Input: part model. Units: mm. Frame: model coordinates. A direction names the side the tool comes from. Coordinates: 2 decimals unless noted, no trailing zeros. Write each loop counter-clockwise with the first axis right and the second up, starting at its lowest first coordinate (ties: lowest second). Pieces come first, ordered by that corner, then holes. Notation, with made-up numbers: M 55,9.25 L 81,9.25 A28 cw 81,40.25 Z; hole C 53.25,70.25 d1. An arc over 180 degrees is marked long. Use one line per item in the form item = value.
from build123d import *

# Parameters (mm, degrees)
BOSS_EXTRUDE1_DEPTH = 100
CUT_EXTRUDE3_REACH  = 138.159
FILLET2_R           = 20
SKETCH6_R           = 4
CUT_EXTRUDE4_DEPTH  = 15


with BuildPart() as part:
    # Sketch1 → Boss-Extrude1 (new body)
    with BuildSketch(Plane.YZ):
        with BuildLine():
            Line((-12.5, 0), (-12.5, -8))
            Line((-12.5, -8), (-10.019077862, -8))
            ThreePointArc((-10.019077862, -8), (-7.561621729, -9.279270691), (-7.2, -12.02606043))
            Line((-7.2, -12.02606043), (-32.25, -80.850369787))
            Line((-32.25, -80.850369787), (-18.415688958, -80.850369787))
            Line((-18.415688958, -80.850369787), (7.381221952, -9.97393957))
            ThreePointArc((7.381221952, -9.97393957), (8.479570506, -8.542543867), (10.200299815, -8))
            Line((10.200299815, -8), (12.5, -8))
            Line((12.5, -8), (12.5, 0))
            Line((12.5, 0), (-12.5, 0))
        make_face()
    extrude(amount=-BOSS_EXTRUDE1_DEPTH)

    # Cut-Extrude3: up to this plane
    cut_extrude3_end = Plane(origin=(-100, -7.2, -12.02606043), z_dir=(0, -0.9396926207859074, 0.34202014332567165))
    # Sketch5 → Cut-Extrude3 (cut, up to the surface)
    with BuildSketch(Plane(origin=(0, 12.5, 0), x_dir=(-1, 0, 0), z_dir=(0, 1, 0)), mode=Mode.PRIVATE) as cut_extrude3_sk1:
        with BuildLine():
            Line((10, -15), (10, -60.850369787))
            ThreePointArc((10, -60.850369787), (12.928932188, -67.921437599), (20, -70.850369787))
            Line((20, -70.850369787), (80, -70.850369787))
            ThreePointArc((80, -70.850369787), (87.071067812, -67.921437599), (90, -60.850369787))
            Line((90, -60.850369787), (90, -15))
            Line((90, -15), (10, -15))
        make_face()
    cut_extrude3_tool1 = split(extrude(cut_extrude3_sk1.sketch, amount=-CUT_EXTRUDE3_REACH, mode=Mode.PRIVATE), bisect_by=cut_extrude3_end, keep=Keep.BOTH, mode=Mode.PRIVATE)
    add(cut_extrude3_tool1.solids().sort_by_distance((-50, 12.5, -42.675996))[0], mode=Mode.SUBTRACT)

    # Fillet2
    fillet2_edges = [part.edges().sort_by_distance(p)[0] for p in [
        (0, -25.332844479, -80.850369787),
        (-100, -25.332844479, -80.850369787),
    ]]
    fillet(fillet2_edges, radius=FILLET2_R)

    # Sketch6 → Cut-Extrude4 (cut)
    with BuildSketch(Plane.XY):
        with Locations((-75, 0)):
            Circle(SKETCH6_R)
        with Locations((-25, 0)):
            Circle(SKETCH6_R)
    extrude(amount=-CUT_EXTRUDE4_DEPTH, mode=Mode.SUBTRACT)


solid = part.part
(1) Pull-direction query (Y, two-part tool) for faces 1 (the flat face through (-49, -11, -8)), 2 (the cylindrical face through (-79, 0, -7)), 3 (the cylindrical face through (-28.2, -2.4, -7.4)), 4 (the cylindrical face through (-49.3, 8.459, -8.557)); classes: pulls with the +Y half, pulls with the -Y half, needs draft (parallel to the pull), parting line crosses it, or undercut.
Computed:
face_1 = needs draft
face_2 = undercut
face_3 = undercut
face_4 = pulls with the +Y half
(2) Section query B-B on y = 0. Return the cut outline in (x, z), plus the area to 3 significant figures.
Computed:
outline = M -100,-30.25 L -90,-30.25 L -90,-15 L -79,-15 L -79,0 L -100,0 Z; M -71,-15 L -29,-15 L -29,0 L -71,0 Z; M -21,-15 L -10,-15 L -10,-30.25 L 0,-30.25 L 0,0 L -21,0 Z
area = 1,570 mm^2
(3) Set-up query: faces 5 (the flat face through (-49, -12.5, -4)), 6 (the flat face through (-46.063, -28.944, -71.768)), 7 (the flat face through (-50, -22, -70.85)). Return all of +Z, -Z, +X, -X, +Y, -Y with unobstructed straight access to the full face (end or side cutting, diameter ignored); none if empty.
Computed:
face_5 = +Z, +X, -X, -Y
face_6 = +X, -X, -Y
face_7 = +Z, +Y, -Y
(4) Section query A-A on x = -54. Return the cut outline in (y, z), plus the area to 3 significant figures.
Computed:
outline = M -32.25,-80.85 L -18.42,-80.85 L -14.78,-70.85 L -28.61,-70.85 Z; M -12.5,-8 L -10.02,-8 A3 cw -7.2,-12.03 L -8.28,-15 L 5.55,-15 L 7.38,-9.97 A3 cw 10.2,-8 L 12.5,-8 L 12.5,0 L -12.5,0 Z
area = 440 mm^2
(5) First-contact query: pin 1 Ø7 at (x, y) = (-60.5, -5) entering from -Z; pin 2 Ø7 at (x, y) = (-62.5, -24.5) entering from +Z; pin 3 Ø2.5 at (x, y) = (-38, -11.5) entering from -Z. Flat tips, straight axial feed; report the tip coordinate or a pass-through.
Computed:
pin_1 = -15
pin_2 = -70.85
pin_3 = -8
(6) Line query: probe 1 along X at (y, z) = (-11, -37.5); probe 2 along Y at (x, z) = (-25, -5.25); probe 3 along Z at (x, y) = (-53, -24). Output: solid intervals per line, ascending.
Computed:
probe_1 = -100 to -90, -10 to 0
probe_2 = -12.5 to -4, 4 to 12.5
probe_3 = -80.85 to -70.85
(7) Section query C-C on x = -25. Return the cut outline in (y, z).
Computed:
outline = M -32.25,-80.85 L -18.42,-80.85 L -14.78,-70.85 L -28.61,-70.85 Z; M -12.5,-8 L -10.02,-8 A3 cw -7.2,-12.03 L -8.28,-15 L -4,-15 L -4,0 L -12.5,0 Z; M 4,-15 L 5.55,-15 L 7.38,-9.97 A3 cw 10.2,-8 L 12.5,-8 L 12.5,0 L 4,0 Z
(8) Section query D-D on z = -36. Return the cut outline in (x, y).
Computed:
outline = M -100,-15.93 L -90,-15.93 L -90,-2.09 L -100,-2.09 Z; M -10,-15.93 L 0,-15.93 L 0,-2.09 L -10,-2.09 Z
